Could you check a few things on this model? Use its own coordinates, in mm. Face numbers are marked on the shaded views. A direction names the side the tool comes from. Give positions to 0.01 mm unless a question says otherwise; leave off trailing zeros. Order: outer loops, then holes, each group sorted by start corner. A loop starts at its lowest first (then second) coordinate and runs counter-clockwise, first axis right, second up. Notation, with made-up numbers: (-8.75, -29.75) -> (41.25, -29.75) arc R16 cw to (41.25, -1.75) -> close; hole circle Ø7 at (45, 70). An arc over 180 degrees is marked (long way). Answer as CSV lines item,"result". Start each with the question number.
(1) On a 3-axis mill with a long thin cutter (end or side, diameter ignored), from which of +Z, -Z, +X, -X, +Y, -Y can I reach the whole of each face in a straight line? I mean the marked faces 1, 2, 3, 4 and 5. Say none if no direction works.
(2) Will these pins go through, and if not, where does the flat tip stop? pin 1 Ø10 at (y, z) = (68, 19) entering from +X; pin 2 Ø11 at (x, y) = (-2.34, 55.52) entering from +Z.
(3) I want a section at A-A (y = 70). Please give me the cut outline in (x, z), plus the area to 3 significant figures.
(4) I want a section at C-C (y = 52). Please give me the cut outline in (x, z).
(5) I need wall thicknesses on L1, parallel to Z at x = 8.5, y = 48; L2, parallel to Z at x = -5.75, y = 75.5; L3, parallel to Z at x = -2.25, y = 42. Which ranges of each line are inside material? Lowest first, please.
(6) I want a section at B-B (x = 7.75). Please give me the cut outline in (y, z), plus the area to 3 significant figures.
(7) We'd pull the mould along Z, two halves only. Please class the marked faces 6, 7, 8 and 9: released by +Z, released by -Z, zero draft, split by the parting line, or undercut.
(8) I want a section at D-D (x = -8.5). Please give me the cut outline in (y, z).
```python
from build123d import *

# Parameters (mm, degrees)
SKETCH1_W                        = 25.4
SKETCH1_H                        = 50.8
BOSS_EXTRUDE1_DEPTH              = 76.2
SKETCH2_W                        = 10.16
SKETCH2_H                        = 38.1
CUT_EXTRUDE1_DEPTH               = 115.016182683
TAP_DRILL_FOR_M16X2_0_TAP2_D     = 14
TAP_DRILL_FOR_M16X2_0_TAP2_DEPTH = 12.7
TAP_DRILL_FOR_M16X2_0_TAP1_D     = 14
TAP_DRILL_FOR_M16X2_0_TAP1_DEPTH = 12.7
FILLET1_R                        = 5


with BuildPart() as part:
    # Sketch1 → Boss-Extrude1 (new body)
    with BuildSketch(Plane.XY):
        with Locations((-2.344226023, 55.520268868)):
            Rectangle(SKETCH1_W, SKETCH1_H)
    extrude(amount=BOSS_EXTRUDE1_DEPTH)

    # Sketch2 → Cut-Extrude1 (cut, through all)
    with BuildSketch(Plane.ZY.offset(15.044226023)):
        with Locations((17.78, 61.870268868)):
            Rectangle(SKETCH2_W, SKETCH2_H)
        with Locations((58.42, 49.170268868)):
            Rectangle(SKETCH2_W, SKETCH2_H)
    extrude(amount=-CUT_EXTRUDE1_DEPTH, mode=Mode.SUBTRACT)

    # Tap Drill for M16x2.0 Tap2
    with Locations(Plane(origin=(0, 0, 0), x_dir=(-1, 0, 0), z_dir=(0, 0, -1))):
        with Locations((2.344226023, 55.520268868)):
            Hole(TAP_DRILL_FOR_M16X2_0_TAP2_D / 2, depth=TAP_DRILL_FOR_M16X2_0_TAP2_DEPTH)

    # Tap Drill for M16x2.0 Tap1
    with Locations(Plane.XY.offset(76.2)):
        with Locations((-2.344226023, 55.520268868)):
            Hole(TAP_DRILL_FOR_M16X2_0_TAP1_D / 2, depth=TAP_DRILL_FOR_M16X2_0_TAP1_DEPTH)

    # Fillet1
    fillet1_edges = [part.edges().sort_by_distance(p)[0] for p in [
        (-2.344226023, 42.820268868, 12.7),
        (-2.344226023, 42.820268868, 22.86),
        (-2.344226023, 68.220268868, 53.34),
        (-2.344226023, 68.220268868, 63.5),
    ]]
    fillet(fillet1_edges, radius=FILLET1_R)


solid = part.part
```
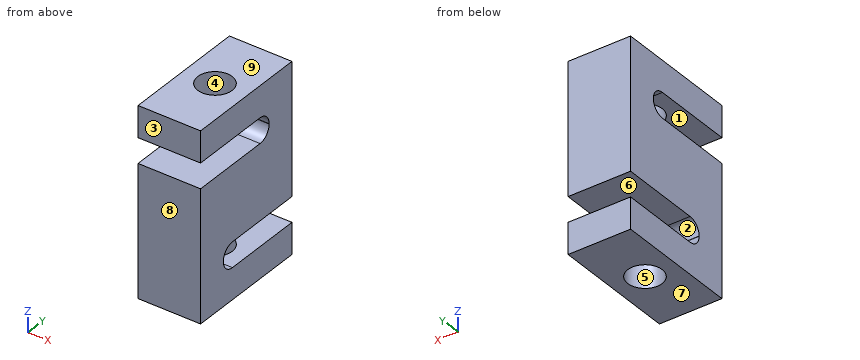
Final values:
1,face 1,"+X, -X, -Y"
1,face 2,"+X, -X, +Y"
1,face 3,"+Z, -Z, +X, -X, -Y"
1,face 4,"+Z"
1,face 5,"-Z"
2,pin 1,"x = 10.36"
2,pin 2,"z = 53.34"
3,outline,"(-15.04, 0) -> (10.36, 0) -> (10.36, 12.7) -> (-15.04, 12.7) -> close; (-15.04, 22.86) -> (10.36, 22.86) -> (10.36, 76.2) -> (-15.04, 76.2) -> close"
3,area,"1,680 mm²"
4,outline,"(-15.04, 0) -> (-8.39, 0) -> (-8.39, 12.7) -> (-15.04, 12.7) -> close; (-15.04, 22.86) -> (10.36, 22.86) -> (10.36, 53.34) -> (-15.04, 53.34) -> close; (-15.04, 63.5) -> (-8.39, 63.5) -> (-8.39, 76.2) -> (-15.04, 76.2) -> close; (3.71, 0) -> (10.36, 0) -> (10.36, 12.7) -> (3.71, 12.7) -> close; (3.71, 63.5) -> (10.36, 63.5) -> (10.36, 76.2) -> (3.71, 76.2) -> close"
5,L1,"0 to 12.7, 22.86 to 53.34, 63.5 to 76.2"
5,L2,"0 to 12.7, 22.86 to 76.2"
5,L3,"0 to 53.34, 63.5 to 76.2"
6,outline,"(30.12, 0) -> (80.92, 0) -> (80.92, 12.7) -> (47.82, 12.7) arc R5 cw to (42.82, 17.7) -> (42.82, 17.86) arc R5 cw to (47.82, 22.86) -> (80.92, 22.86) -> (80.92, 76.2) -> (30.12, 76.2) -> (30.12, 63.5) -> (63.22, 63.5) arc R5 cw to (68.22, 58.5) -> (68.22, 58.34) arc R5 cw to (63.22, 53.34) -> (30.12, 53.34) -> close"
6,area,"3,120 mm²"
7,face 6,"undercut"
7,face 7,"released by -Z"
7,face 8,"zero draft"
7,face 9,"released by +Z"
8,outline,"(30.12, 0) -> (52.19, 0) -> (52.19, 12.7) -> (47.82, 12.7) arc R5 cw to (42.82, 17.7) -> (42.82, 17.86) arc R5 cw to (47.82, 22.86) -> (80.92, 22.86) -> (80.92, 76.2) -> (58.85, 76.2) -> (58.85, 63.5) -> (63.22, 63.5) arc R5 cw to (68.22, 58.5) -> (68.22, 58.34) arc R5 cw to (63.22, 53.34) -> (30.12, 53.34) -> close; (30.12, 63.5) -> (52.19, 63.5) -> (52.19, 76.2) -> (30.12, 76.2) -> close; (58.85, 0) -> (80.92, 0) -> (80.92, 12.7) -> (58.85, 12.7) -> close"
